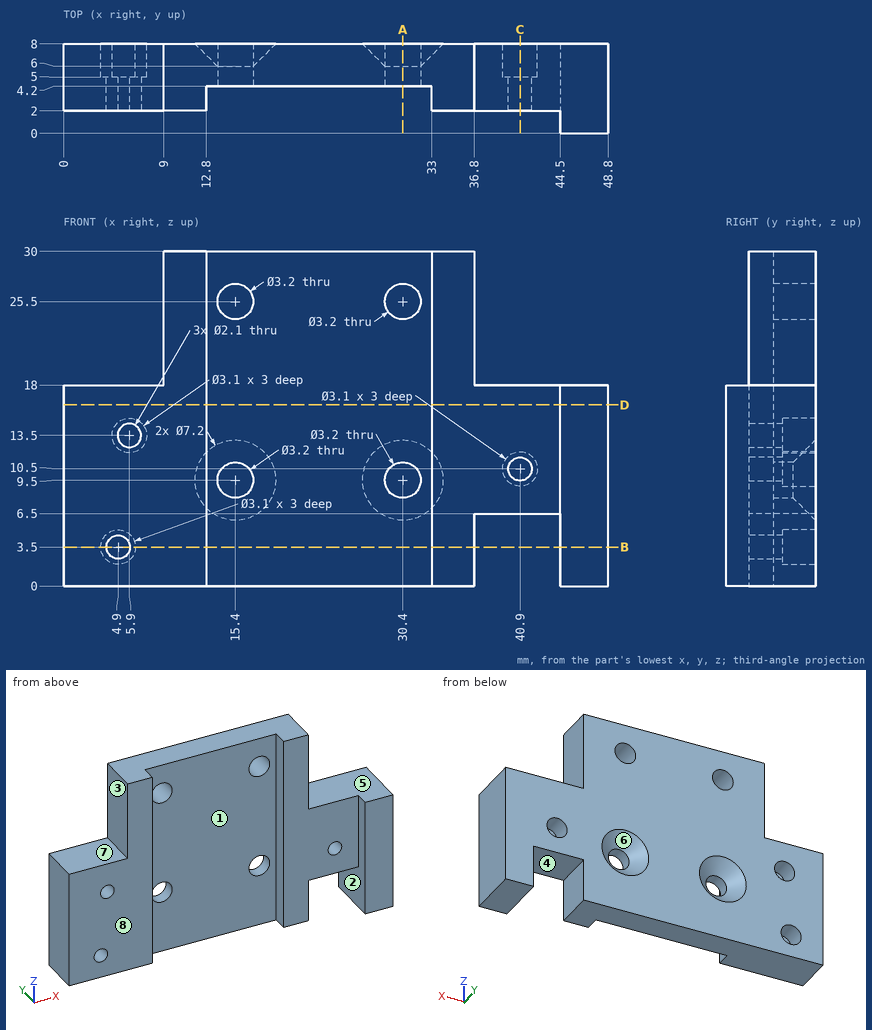
The drawing under review shows one solid part. Ordinate dimensions are in mm from its lowest x, y, z. A direction names the side the tool comes from. Coordinates: 2 decimals unless noted, no trailing zeros. Write each loop counter-clockwise with the first axis right and the second up, starting at its lowest first coordinate (ties: lowest second). Pieces come first, ordered by that corner, then holes. Notation, with made-up numbers: (34, 26.5) - (78, 26.5) arc R27 ccw to (78, 65.5) - close; hole circle Ø9 at (69, 76.5). An arc over 180 degrees is marked (long way). Put each result on its own line as item: value.
1. Mouldability with a two-part tool opening along Z and no side actions: class the marked faces 6, 7 and 8 as released by +Z, released by -Z, zero draft, split by the parting line, or undercut.
Values found:
face 6: undercut
face 7: released by +Z
face 8: zero draft
2. For pin 1 (2 mm diameter, centred on x = 42, y = 1.5, fed in from +Z); pin 2 (3 mm diameter, centred on x = 15.4, z = 9.5, fed in from +Y); pin 3 (0.9 mm diameter, centred on x = 5.5, z = 3, fed in from +Y); pin 4 (2 mm diameter, centred on x = 37, z = 23, fed in from -Y), all flat-tipped, find the tip position at first contact; note any pin that passes through.
Values found:
pin 1: z = 18
pin 2: through
pin 3: y = 5
pin 4: y = 2
3. Add section A-A, the plane x = 30.4. Give the boundary of the cut face in (y, z), then the cut area to 3 significant figures.
Values found:
outline: (4.2, 0) - (8, 0) - (8, 5.9) - (6, 7.9) - (4.2, 7.9) - close; (4.2, 11.1) - (6, 11.1) - (8, 13.1) - (8, 23.9) - (4.2, 23.9) - close; (4.2, 27.1) - (8, 27.1) - (8, 30) - (4.2, 30) - close
area: 85.7 mm²
4. Machinability: for the marked faces 1, 2, 3, 4 and 5, which of the approach directions +Z, -Z, +X, -X, +Y, -Y give a long, thin tool a straight path to every point of the face, cutting with its end or side? Answer none if there is none.
Values found:
face 1: +Z, -Z, -Y
face 2: -Z, -Y
face 3: +Z, -X, +Y, -Y
face 4: -Z, +Y, -Y
face 5: +Z, +X, +Y, -Y
5. Add section B-B, the plane z = 3.5. Give the boundary of the cut face in (x, y).
Values found:
outline: (0, 2) - (3.85, 2) - (3.85, 5) - (3.35, 5) - (3.35, 8) - (0, 8) - close; (5.95, 2) - (12.8, 2) - (12.8, 4.2) - (33, 4.2) - (33, 2) - (36.8, 2) - (36.8, 8) - (6.45, 8) - (6.45, 5) - (5.95, 5) - close; (44.5, 0) - (48.8, 0) - (48.8, 8) - (44.5, 8) - close
6. Add section C-C, the plane x = 40.9. Give the boundary of the cut face in (y, z).
Values found:
outline: (2, 6.5) - (8, 6.5) - (8, 8.95) - (5, 8.95) - (5, 9.45) - (2, 9.45) - close; (2, 11.55) - (5, 11.55) - (5, 12.05) - (8, 12.05) - (8, 18) - (2, 18) - close
7. Add section D-D, the plane z = 16.25. Give the boundary of the cut face in (x, y).
Values found:
outline: (0, 2) - (12.8, 2) - (12.8, 4.2) - (33, 4.2) - (33, 2) - (44.5, 2) - (44.5, 0) - (48.8, 0) - (48.8, 8) - (0, 8) - close
8. Wall thickness on probe 1 along X at (y, z) = (3.5, 28.5); probe 2 along X at (y, z) = (5.8, 25.5); probe 3 along X at (y, z) = (2.85, 3.5): over which ranges is each line inside the solid? List them lowest first.
Values found:
probe 1: 9 to 12.8, 33 to 36.8
probe 2: 9 to 13.8, 17 to 28.8, 32 to 36.8
probe 3: 0 to 3.85, 5.95 to 12.8, 33 to 36.8, 44.5 to 48.8
